```python
from build123d import *

# Parameters (mm, degrees)
SKETCH1_W           = 40
SKETCH1_H           = 7
BOSS_EXTRUDE1_DEPTH = 55
SKETCH2_R           = 2.684543284
CUT_EXTRUDE1_DEPTH  = 7
FILLET1_RADIUS      = 20
FILLET1_LENGTH      = 7
SKETCH4_W           = 20
SKETCH4_H           = 5
CUT_EXTRUDE2_DEPTH  = 40


with BuildPart() as part:
    # Sketch1 → Boss-Extrude1 (new body)
    with BuildSketch(Plane.XY):
        with Locations((20, -3.5)):
            Rectangle(SKETCH1_W, SKETCH1_H)
    extrude(amount=BOSS_EXTRUDE1_DEPTH)

    # Sketch2 → Cut-Extrude1 (cut)
    with BuildSketch(Plane(origin=(0, 0, 0), x_dir=(1, 0, 0), z_dir=(0, 1, 0))):
        with Locations(Location((20, -10, 0), (0, 0, 270))):
            Circle(SKETCH2_R)
        with Locations(Location((20, -20, 0), (0, 0, 270))):
            Circle(SKETCH2_R)
        with Locations(Location((20, -30, 0), (0, 0, 270))):
            Circle(SKETCH2_R)
    extrude(amount=-CUT_EXTRUDE1_DEPTH, mode=Mode.SUBTRACT)

    # Fillet1: full round fillet: the end face becomes a half cylinder, R = half its width
    fillet1_face = Plane((20, -3.5, 55), x_dir=(0, 1, 0), z_dir=(0, 0, 1))  # on the end face: x along it, z out of the body
    fillet1_slab = fillet1_face.offset(-FILLET1_RADIUS / 2) * Box(FILLET1_LENGTH, 2 * FILLET1_RADIUS, FILLET1_RADIUS, mode=Mode.PRIVATE)  # the body's end, R deep
    fillet1_round = Plane((20, -3.5, 35), x_dir=(0, 0, 1), z_dir=(0, 1, 0)) * Cylinder(FILLET1_RADIUS, FILLET1_LENGTH, mode=Mode.PRIVATE)  # its axis R under the face
    add(fillet1_slab - fillet1_round, mode=Mode.SUBTRACT)

    # Sketch4 → Cut-Extrude2 (cut)
    with BuildSketch(Plane(origin=(0, 0, 0), x_dir=(-1, 0, 0), z_dir=(0, 0, -1))):
        with Locations((-20, -3.5)):
            Rectangle(SKETCH4_W, SKETCH4_H)
    extrude(amount=-CUT_EXTRUDE2_DEPTH, mode=Mode.SUBTRACT)


solid = part.part
```
Build history of the part. All positions in model axes, mm. A direction names the side the tool comes from. Give positions to 0.01 mm unless a question says otherwise; leave off trailing zeros. Loops run counter-clockwise (first coordinate to the right, second up) from the corner with the lowest first, then second, coordinate; pieces in that order, holes last.
1) 3-axis set-ups, long thin cutter, end or side, ignore diameter. For faces 4 (the face through (10, -4, 20)), 5 (the face through (20.12, -6.49, 27.32)): which of +Z, -Z, +X, -X, +Y, -Y reach the whole face in a straight line?
Values follow:
face 4: -Z
face 5: +Y, -Y
2) Two-plate mould, pull along X, no slides. Class faces 1 (the face through (20, -3, 40)), 2 (the face through (19.7, -6.6, 0)), 3 (the face through (20, -3, 55)): released by +X, released by -X, zero draft, split by the parting line, or undercut.
Values follow:
face 1: undercut
face 2: zero draft
face 3: split by the parting line
3) Band-saw the part on B-B on x = 20. State how many separate pieces and enclosed holes the cut face has, then the cut area to 3 significant figures.
Values follow:
separate pieces: 7
enclosed holes: 0
area: 153 mm2
4) Band-saw the part on A-A on z = 6.5. List the corners of the cut face in (x, y), then the cut area to 3 significant figures.
Values follow:
outline: (0, -7) - (40, -7) - (40, 0) - (0, 0) - close; hole (10, -6) - (30, -6) - (30, -1) - (10, -1) - close
area: 180 mm2
5) Probe line 1 along X through (y, z) = (-1.25, 33.5); line 2 along X through (y, z) = (-0.8, 30); line 3 along Y through (x, z) = (17.5, 6). List the from-to ranges inside material, lowest first.
Values follow:
line 1: x = 0 to 10, 30 to 40
line 2: x = 0 to 17.32, 22.68 to 40
line 3: y = -7 to -6, -1 to 0
6) Drop a flat-ended pin along its axis: P1, Ø3, axis at y = -1.5, z = 48.5, coming from the +X side. Give the stop position or say it passes through.
Values follow:
P1: stops at x = 36
7) Band-saw the part on D-D on z = 29.5. List the corners of the cut face in (x, y), then the cut area to 3 significant figures.
Values follow:
outline: (0, -7) - (17.36, -7) - (17.36, -6) - (10, -6) - (10, -1) - (17.36, -1) - (17.36, 0) - (0, 0) - close; (22.64, -7) - (40, -7) - (40, 0) - (22.64, 0) - (22.64, -1) - (30, -1) - (30, -6) - (22.64, -6) - close
area: 169 mm2
8) Band-saw the part on C-C on y = -2.5. List the corners of the cut face in (x, z).
Values follow:
outline: (0, 0) - (10, 0) - (10, 40) - (30, 40) - (30, 0) - (40, 0) - (40, 35) arc R20 ccw to (0, 35) - close
